Job drawing, mm, ordinate dimensions from the low corner. One solid piece. A direction names the side the tool comes from. Coordinates: 2 decimals unless noted, no trailing zeros. Order: outer loops, then holes, each group sorted by start corner. A loop starts at its lowest first (then second) coordinate and runs counter-clockwise, first axis right, second up. Notation, with made-up numbers: M -30.75,20 L -26.75,20 A28 cw -26.75,57 Z; hole C 61,-28.75 d4. An arc over 180 degrees is marked long. Write item = value, one per line. Start each with the question number.
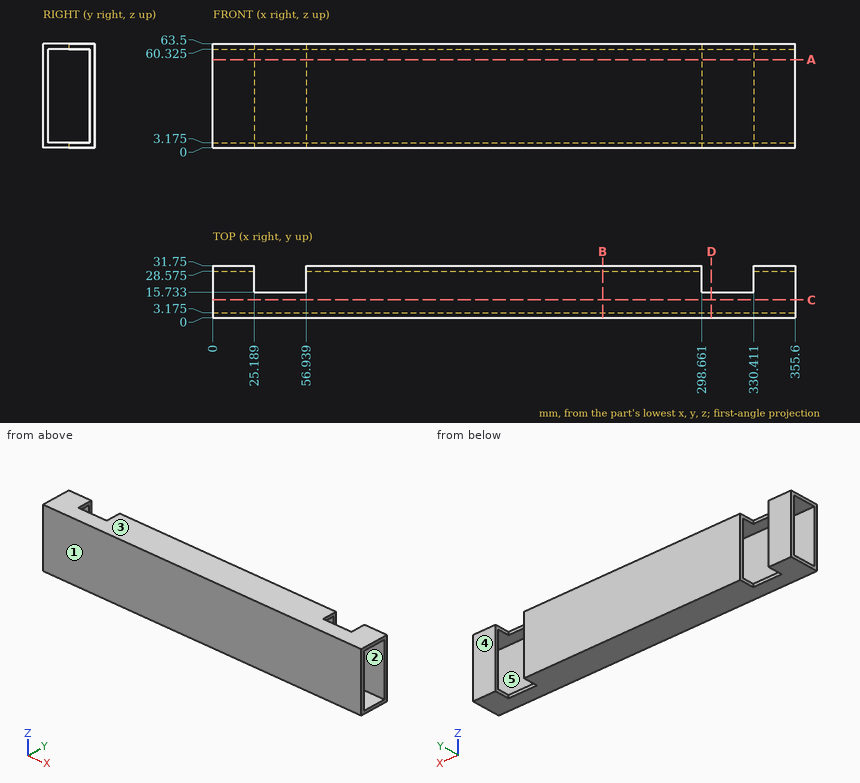
Item 1: Cut at B-B, the plane x = 238. Write the cut outline in (y, z) (3 decimals).
Item 2: Cut at C-C, the plane y = 11. Write the cut outline in (x, z) (3 decimals).
Item 3: Flat gauge pins, fed straight in: pin 1 (1.6 mm diameter, centred on x = 322, z = 1.5, fed in from +Y); pin 2 (2 mm diameter, centred on x = 53.5, z = 36.5, fed in from +Y) (3 decimals). Where does each tip first touch, or does it go through?
Item 4: Cut at D-D, the plane x = 304.5. Write the cut outline in (y, z) (1 decimal).
Item 5: Wall check: line 1 along X through (y, z) = (30.5, 26.5); line 2 along Z through (x, y) = (334, 22) (3 decimals); line 3 along Y through (x, z) = (223, 48) (3 decimals). Give the ranges that are in metal, low to high. Write a range as [from, to].
Item 6: Pull direction Z, two halves, no side cores. Call the marked faces 3, 4 and 5: pulls with the +Z half, pulls with the -Z half, needs draft (parallel to the pull), parting line crosses it, or undercut.
Item 7: Cut at A-A, the plane z = 54. Count the separate pieces of the cut face and the enclosed holes in it, and give its area (3 significant figures).
Item 8: 3-axis set-ups, long thin cutter, end or side, ignore diameter. For the marked faces 1 and 2: which of +Z, -Z, +X, -X, +Y, -Y reach the whole face in a straight line?
Filled sheet:
q1.outline = M 0,0 L 31.75,0 L 31.75,63.5 L 0,63.5 Z; hole M 3.175,3.175 L 28.575,3.175 L 28.575,60.325 L 3.175,60.325 Z
q2.outline = M 0,0 L 355.6,0 L 355.6,3.175 L 0,3.175 Z; M 0,60.325 L 355.6,60.325 L 355.6,63.5 L 0,63.5 Z
q3.pin_1 = 15.73
q3.pin_2 = 3.175
q4.outline = M 0,0 L 15.7,0 L 15.7,3.2 L 3.2,3.2 L 3.2,60.3 L 15.7,60.3 L 15.7,63.5 L 0,63.5 Z
q5.line_1 = [0, 25.19], [56.94, 298.66], [330.41, 355.6]
q5.line_2 = [0, 3.175], [60.325, 63.5]
q5.line_3 = [0, 3.175], [28.575, 31.75]
q6.face_3 = pulls with the +Z half
q6.face_4 = needs draft
q6.face_5 = undercut
q7.separate_pieces = 4
q7.enclosed_holes = 0
q7.area = 2,060 mm2
q8.face_1 = +Z, -Z, +X, -X, -Y
q8.face_2 = +X, -X
